The model under review builds one solid part; all positions refer to its coordinate system, in mm. Face numbers are marked on the shaded views. A direction names the side the tool comes from. Round coordinates to 2 decimals unless told otherwise and drop trailing zeros. Loops run counter-clockwise (first coordinate to the right, second up) from the corner with the lowest first, then second, coordinate; pieces in that order, holes last. Notation, with made-up numbers: M 66,22 L 71,22 A23 cw 71,34 Z; hole C 78.5,14.5 d3. An arc over 180 degrees is marked long. Return JSON: item names as keys, results as strings. Group by question number.
Q1. For the marked faces 1, 2 and 3, list the 3-axis set-ups (+Z, -Z, +X, -X, +Y, -Y) from which the entire face can be reached by the end or side of a thin tool; tool diameter is ignored.
Q2. Draft analysis for pull direction X (two halves, no side actions). For the marked faces 4, 5 and 6, state which applies: pulls with the +X half, pulls with the -X half, needs draft (parallel to the pull), parting line crosses it, or undercut.
Q3. Consider section B-B (x = 60). State the section outline as (y, z) points.
Q4. Consider section C-C (x = 72). State the section outline as (y, z) points, and give its area (3 significant figures).
Q5. Clearance check with flat-ended pins moving along their axes: pin 1 Ø2 at (x, z) = (69.5, 12.5) entering from -Y; pin 2 Ø12 at (x, z) = (62, 5) entering from +Y; pin 3 Ø12 at (y, z) = (18.5, 8) entering from +X; pin 4 Ø2.5 at (x, y) = (60, 5) entering from +Z. State where each tip first meets the part, or that it passes through.
Q6. Consider section D-D (y = 19.5). State the section outline as (x, z) points, and give its area (3 significant figures).
Q7. To check wall thickness, follow line 1 along Y through (x, z) = (60, 1.45); line 2 along Z through (x, y) = (69, 23); line 3 along X through (y, z) = (9.5, 7.5). State the ranges of each line that lie inside material, in increasing order.
Q8. Consider section A-A (y = 5). State the section outline as (x, z) points, and give its area (3 significant figures).
Autodesk Inventor part; units mm, degrees
ref_plane "YZ Plane" through (0, 0, 0) normal (1, 0, 0) x (0, 1, 0)
ref_plane "XZ Plane" through (0, 0, 0) normal (0, 1, 0) x (-1, 0, 0)
ref_plane "XY Plane" through (0, 0, 0) normal (0, 0, 1) x (1, 0, 0)
sketch "Эскиз1" plane through (0, 0, 0) normal (0, 0, 1) x (1, 0, 0)
  line L0 (0, 80) -> (80, 0)
  line L1 (2.2627, 82.2627) -> (82.2627, 2.2627)
  line L2 (0, 80) -> (2.2627, 82.2627)
  line L3 (80, 0) -> (82.2627, 2.2627)
  point P0 (0, 0)
  dimension "d2" = 3.2
extrude "Выдавливание1" add sketch "Эскиз1" along normal blind 38.75
sketch "Эскиз2" plane through (0, 0, 0) normal (0, 0, -1) x (-1, 0, 0)
  line L0 (0, 80) -> (-80, 0)
  line L1 (-55, 25) -> (-55, -25)
  line L2 (-80, 0) -> (-55, 0)
  line L3 (-55, 8) -> (-60, 8)
  line L4 (-60, 8) -> (-60, 33)
  circle A0 centre (-60, 12) radius 2
  circle A1 centre (-60, 5) radius 2
  point P0 (0, 0)
  dimension "d5" = 4
extrude "Выдавливание2" add sketch "Эскиз2" against normal blind 3 contours L1 L3 L4 A0 L0 | L4 A0 L3 L1 L2 L0
sketch "Эскиз3" plane through (2.2627, 82.2627, 0) normal (0.7071068, 0.7071068, 0) x (-0.7071068, 0.7071068, 0)
  line L0 (-113.1371, 0) -> (-95.4594, 0)
  line L1 (0, 38.75) -> (-113.1371, 38.75)
  line L2 (-113.1371, 0) -> (-110.1371, 0)
  line L3 (-110.1371, 0) -> (-110.1371, 38.75)
  line L4 (-110.1371, 38.75) -> (-113.1371, 38.75)
  line L5 (-113.1371, 38.75) -> (-113.1371, 0)
  point P0 (-56.5685, 0)
  point P1 (-113.1371, 38.75)
  dimension "d8" = 3
extrude "Выдавливание3" add sketch "Эскиз3" along normal blind 4.5
sketch "Эскиз4" plane through (5.4447, 85.4447, 0) normal (0.7071068, 0.7071068, 0) x (0, 0, 1)
  line L0 (0, 113.1371) -> (3, 113.1371)
  line L1 (0, 0) -> (38.75, 0)
  line L2 (0, 113.1371) -> (7, 113.1371)
  line L3 (7, 113.1371) -> (7, 0)
  line L4 (7, 0) -> (0, 0)
  line L5 (0, 0) -> (0, 113.1371)
  line L6 (38.75, 0) -> (38.75, 113.1371)
  line L7 (7, 113.1371) -> (38.75, 113.1371)
  line L8 (38.75, 113.1371) -> (38.75, 105)
  line L9 (38.75, 105) -> (7, 105)
  line L10 (7, 105) -> (7, 113.1371)
  point P0 (0, 56.5685)
  point P1 (38.75, 113.1371)
  point P2 (7, 105)
extrude "Выдавливание4" add sketch "Эскиз4" along normal blind 3 contours L0 L2 L3 L1 L5 | L7 L6 L9 L3
sketch "Эскиз5" plane through (0, 0, 0) normal (0, 0, -1) x (-1, 0, 0)
  line L0 (-80.1414, 4.3841) -> (-2.2627, 82.2627)
  circle A0 centre (-60, 12) radius 2
  circle A1 centre (-60, 5) radius 2
  line L1 (0, 80) -> (-55, 25)
  line L2 (-2.2627, 82.2627) -> (0, 80)
  line L3 (-80.1414, 4.3841) -> (-2.2627, 82.2627)
  line L4 (-80.1414, 4.3841) -> (-83.3234, 7.566)
  line L5 (-83.3234, 7.566) -> (-5.4447, 85.4447)
  line L6 (-5.4447, 85.4447) -> (-7.566, 87.566)
  line L7 (-87.566, 7.566) -> (-7.566, 87.566)
  line L8 (-80, 0) -> (-87.566, 7.566)
  line L9 (-80, 0) -> (-55, 0)
  line L10 (-55, 0) -> (-55, 25)
  line L11 (-5.4447, 85.4447) -> (-2.2627, 82.2627)
  line L12 (-83.3234, 7.566) -> (-5.4447, 85.4447)
  point P0 (0, 0)
  point P1 (-2.2627, 82.2627)
extrude "Выдавливание5" add sketch "Эскиз5" against normal blind 3 contours L4 L5 L11 L0
sketch "Эскиз6" plane through (7.566, 87.566, 0) normal (0.7071068, 0.7071068, 0) x (-0.7071068, 0.7071068, 0)
  line L0 (0, 0) -> (-77.7817, 0)
  line L1 (-110.1371, 38.75) -> (0, 38.75)
  line L2 (0, 0) -> (-70, 0)
  line L3 (-70, 0) -> (-70, 38.75)
  line L4 (-70, 38.75) -> (0, 38.75)
  line L5 (0, 38.75) -> (0, 0)
  line L6 (-81, 0) -> (-81, 51)
  line L7 (-113.1371, 0) -> (0, 0)
  point P0 (-56.5685, 0)
  point P1 (0, 38.75)
  point P2 (-81, 38.75)
extrude "Выдавливание6" cut sketch "Эскиз6" against normal through all
sketch "Эскиз7" plane through (0, 0, 38.75) normal (0, 0, 1) x (1, 0, 0)
  line L0 (59.5384, 24.9871) -> (57.2756, 22.7244)
  line L1 (57.2756, 22.7244) -> (80, 0)
  line L2 (80, 0) -> (87.566, 7.566)
  line L3 (81.8123, 13.3198) -> (87.566, 7.566)
  line L4 (79.6909, 11.1985) -> (81.8123, 13.3198)
  line L5 (79.6909, 11.1985) -> (83.3234, 7.566)
  line L6 (80.1414, 4.3841) -> (83.3234, 7.566)
  line L7 (80.1414, 4.3841) -> (59.5384, 24.9871)
  point P0 (0, 0)
extrude "Выдавливание7" cut sketch "Эскиз7" against normal blind 13
properties part number "фанера"
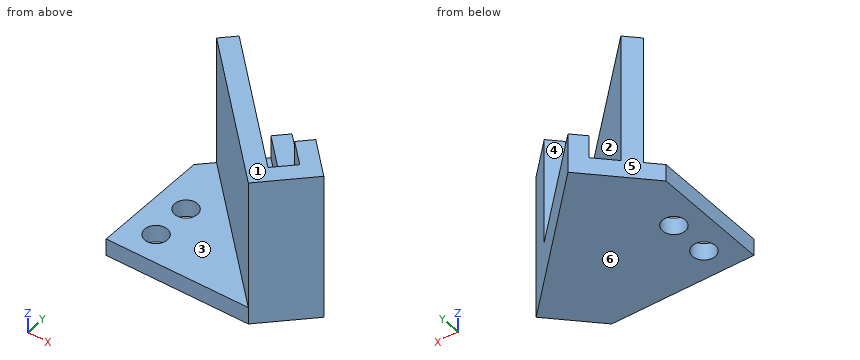
Values:
{
 "1": {"face 1": "+Z, +X, -X, +Y, -Y", "face 2": "+Z", "face 3": "+Z, -X, -Y"},
 "2": {"face 4": "undercut", "face 5": "pulls with the -X half", "face 6": "needs draft"},
 "3": {"outline": "M 0,0 L 3,0 L 3,3 L 0,3 Z; M 7,0 L 10,0 L 10,3 L 7,3 Z; M 14,0 L 25.45,0 L 25.45,3 L 24.53,3 L 24.53,25.75 L 20,25.75 L 20,3 L 14,3 Z"},
 "4": {"outline": "M 0,0 L 23.13,0 L 23.13,7 L 18.89,7 L 18.89,3 L 12.53,3 L 12.53,25.75 L 8,25.75 L 8,3 L 0,3 Z", "area": "189 mm2"},
 "5": {"pin 1": "stops at y = 9.5", "pin 2": "stops at y = 30.29", "pin 3": "stops at x = 82.63", "pin 4": "passes through"},
 "6": {"outline": "M 55,0 L 75.63,0 L 75.63,7 L 71.39,7 L 71.39,3 L 65.03,3 L 65.03,25.75 L 60.5,25.75 L 60.5,3 L 55,3 Z", "area": "182 mm2"},
 "7": {"line 1": "y = 0 to 3, 7 to 10, 14 to 25.45", "line 2": "z = 0 to 7", "line 3": "x = 70.5 to 75.03, 81.39 to 85.63"},
 "8": {"outline": "M 55,0 L 58,0 L 58,3 L 55,3 Z; M 62,0 L 85,0 L 85,25.75 L 80.76,25.75 L 80.76,3 L 79.53,3 L 79.53,25.75 L 75,25.75 L 75,3 L 62,3 Z", "area": "277 mm2"}
}
